Design review of the part built by this model. Coordinates are the model's own, in mm. A direction names the side the tool comes from. Round coordinates to 2 decimals unless told otherwise and drop trailing zeros.
from build123d import *

# Parameters (mm, degrees)
SKETCH_1_R      = 3.4
EXTRUDE_1_DEPTH = 1000


with BuildPart() as part:
    # Эскиз1 → Бобышка-Вытянуть1 (new body)
    with BuildSketch(Plane.XY):
        with BuildLine():
            Line((-20, 15.5), (-20, 10.25))
            Line((-20, 10.25), (-20, 5.4))
            ThreePointArc((-20, 5.4), (-19.912132034, 5.187867966), (-19.7, 5.1))
            Line((-19.7, 5.1), (-19.3, 5.1))
            ThreePointArc((-19.3, 5.1), (-19.087867966, 5.012132034), (-19, 4.8))
            Line((-19, 4.8), (-19, 4.4))
            ThreePointArc((-19, 4.4), (-18.912132034, 4.187867966), (-18.7, 4.1))
            Line((-18.7, 4.1), (-15.8, 4.1))
            ThreePointArc((-15.8, 4.1), (-15.587867966, 4.187867966), (-15.5, 4.4))
            Line((-15.5, 4.4), (-15.5, 6.3))
            ThreePointArc((-15.5, 6.3), (-15.587867966, 6.512132034), (-15.8, 6.6))
            Line((-15.8, 6.6), (-17, 6.6))
            ThreePointArc((-17, 6.6), (-17.707106781, 6.892893219), (-18, 7.6))
            Line((-18, 7.6), (-18, 9.25))
            ThreePointArc((-18, 9.25), (-17.707106781, 9.957106781), (-17, 10.25))
            Line((-17, 10.25), (-12.464213562, 10.25))
            ThreePointArc((-12.464213562, 10.25), (-12.08153013, 10.173879533), (-11.757106781, 9.957106781))
            Line((-11.757106781, 9.957106781), (-7.992893219, 6.192893219))
            ThreePointArc((-7.992893219, 6.192893219), (-7.776120467, 5.86846987), (-7.7, 5.485786438))
            Line((-7.7, 5.485786438), (-7.7, -5.485786438))
            ThreePointArc((-7.7, -5.485786438), (-7.776120467, -5.86846987), (-7.992893219, -6.192893219))
            Line((-7.992893219, -6.192893219), (-11.757106781, -9.957106781))
            ThreePointArc((-11.757106781, -9.957106781), (-12.08153013, -10.173879533), (-12.464213562, -10.25))
            Line((-12.464213562, -10.25), (-17, -10.25))
            ThreePointArc((-17, -10.25), (-17.707106781, -9.957106781), (-18, -9.25))
            Line((-18, -9.25), (-18, -7.6))
            ThreePointArc((-18, -7.6), (-17.707106781, -6.892893219), (-17, -6.6))
            Line((-17, -6.6), (-15.8, -6.6))
            ThreePointArc((-15.8, -6.6), (-15.587867966, -6.512132034), (-15.5, -6.3))
            Line((-15.5, -6.3), (-15.5, -4.4))
            ThreePointArc((-15.5, -4.4), (-15.587867966, -4.187867966), (-15.8, -4.1))
            Line((-15.8, -4.1), (-18.7, -4.1))
            ThreePointArc((-18.7, -4.1), (-18.912132034, -4.187867966), (-19, -4.4))
            Line((-19, -4.4), (-19, -4.8))
            ThreePointArc((-19, -4.8), (-19.087867966, -5.012132034), (-19.3, -5.1))
            Line((-19.3, -5.1), (-19.7, -5.1))
            ThreePointArc((-19.7, -5.1), (-19.912132034, -5.187867966), (-20, -5.4))
            Line((-20, -5.4), (-20, -10.25))
            Line((-20, -10.25), (-20, -15.5))
            ThreePointArc((-20, -15.5), (-18.681980515, -18.681980515), (-15.5, -20))
            Line((-15.5, -20), (-10.25, -20))
            Line((-10.25, -20), (0, -20))
            Line((0, -20), (10.25, -20))
            Line((10.25, -20), (15.5, -20))
            ThreePointArc((15.5, -20), (18.681980515, -18.681980515), (20, -15.5))
            Line((20, -15.5), (20, -10.25))
            Line((20, -10.25), (20, 0))
            Line((20, 0), (20, 10.25))
            Line((20, 10.25), (20, 15.5))
            ThreePointArc((20, 15.5), (18.681980515, 18.681980515), (15.5, 20))
            Line((15.5, 20), (10.25, 20))
            Line((10.25, 20), (5.4, 20))
            ThreePointArc((5.4, 20), (5.187867966, 19.912132034), (5.1, 19.7))
            Line((5.1, 19.7), (5.1, 19.3))
            ThreePointArc((5.1, 19.3), (5.012132034, 19.087867966), (4.8, 19))
            Line((4.8, 19), (4.4, 19))
            ThreePointArc((4.4, 19), (4.187867966, 18.912132034), (4.1, 18.7))
            Line((4.1, 18.7), (4.1, 15.8))
            ThreePointArc((4.1, 15.8), (4.187867966, 15.587867966), (4.4, 15.5))
            Line((4.4, 15.5), (6.3, 15.5))
            ThreePointArc((6.3, 15.5), (6.512132034, 15.587867966), (6.6, 15.8))
            Line((6.6, 15.8), (6.6, 17))
            ThreePointArc((6.6, 17), (6.892893219, 17.707106781), (7.6, 18))
            Line((7.6, 18), (9.25, 18))
            ThreePointArc((9.25, 18), (9.957106781, 17.707106781), (10.25, 17))
            Line((10.25, 17), (10.25, 12.464213562))
            ThreePointArc((10.25, 12.464213562), (10.173879533, 12.08153013), (9.957106781, 11.757106781))
            Line((9.957106781, 11.757106781), (6.192893219, 7.992893219))
            ThreePointArc((6.192893219, 7.992893219), (5.86846987, 7.776120467), (5.485786438, 7.7))
            Line((5.485786438, 7.7), (-5.485786438, 7.7))
            ThreePointArc((-5.485786438, 7.7), (-5.86846987, 7.776120467), (-6.192893219, 7.992893219))
            Line((-6.192893219, 7.992893219), (-9.957106781, 11.757106781))
            ThreePointArc((-9.957106781, 11.757106781), (-10.173879533, 12.08153013), (-10.25, 12.464213562))
            Line((-10.25, 12.464213562), (-10.25, 17))
            ThreePointArc((-10.25, 17), (-9.957106781, 17.707106781), (-9.25, 18))
            Line((-9.25, 18), (-7.6, 18))
            ThreePointArc((-7.6, 18), (-6.892893219, 17.707106781), (-6.6, 17))
            Line((-6.6, 17), (-6.6, 15.8))
            ThreePointArc((-6.6, 15.8), (-6.512132034, 15.587867966), (-6.3, 15.5))
            Line((-6.3, 15.5), (-4.4, 15.5))
            ThreePointArc((-4.4, 15.5), (-4.187867966, 15.587867966), (-4.1, 15.8))
            Line((-4.1, 15.8), (-4.1, 18.7))
            ThreePointArc((-4.1, 18.7), (-4.187867966, 18.912132034), (-4.4, 19))
            Line((-4.4, 19), (-4.8, 19))
            ThreePointArc((-4.8, 19), (-5.012132034, 19.087867966), (-5.1, 19.3))
            Line((-5.1, 19.3), (-5.1, 19.7))
            ThreePointArc((-5.1, 19.7), (-5.187867966, 19.912132034), (-5.4, 20))
            Line((-5.4, 20), (-10.25, 20))
            Line((-10.25, 20), (-15.5, 20))
            ThreePointArc((-15.5, 20), (-18.681980515, 18.681980515), (-20, 15.5))
        make_face()
        with BuildLine():
            ThreePointArc((-12.8, -11.8), (-12.092893219, -12.092893219), (-11.8, -12.8))
            Line((-11.8, -12.8), (-11.8, -17))
            ThreePointArc((-11.8, -17), (-12.092893219, -17.707106781), (-12.8, -18))
            Line((-12.8, -18), (-15.5, -18))
            ThreePointArc((-15.5, -18), (-17.267766953, -17.267766953), (-18, -15.5))
            Line((-18, -15.5), (-18, -12.8))
            ThreePointArc((-18, -12.8), (-17.707106781, -12.092893219), (-17, -11.8))
            Line((-17, -11.8), (-12.8, -11.8))
        make_face(mode=Mode.SUBTRACT)
        with BuildLine():
            Line((9.25, -18), (0, -18))
            Line((0, -18), (-9.25, -18))
            ThreePointArc((-9.25, -18), (-9.957106781, -17.707106781), (-10.25, -17))
            Line((-10.25, -17), (-10.25, -12.464213562))
            ThreePointArc((-10.25, -12.464213562), (-10.173879533, -12.08153013), (-9.957106781, -11.757106781))
            Line((-9.957106781, -11.757106781), (-6.192893219, -7.992893219))
            ThreePointArc((-6.192893219, -7.992893219), (-5.86846987, -7.776120467), (-5.485786438, -7.7))
            Line((-5.485786438, -7.7), (5.485786438, -7.7))
            ThreePointArc((5.485786438, -7.7), (5.86846987, -7.776120467), (6.192893219, -7.992893219))
            Line((6.192893219, -7.992893219), (9.957106781, -11.757106781))
            ThreePointArc((9.957106781, -11.757106781), (10.173879533, -12.08153013), (10.25, -12.464213562))
            Line((10.25, -12.464213562), (10.25, -17))
            ThreePointArc((10.25, -17), (9.957106781, -17.707106781), (9.25, -18))
        make_face(mode=Mode.SUBTRACT)
        with BuildLine():
            ThreePointArc((11.8, -12.8), (12.092893219, -12.092893219), (12.8, -11.8))
            Line((12.8, -11.8), (17, -11.8))
            ThreePointArc((17, -11.8), (17.707106781, -12.092893219), (18, -12.8))
            Line((18, -12.8), (18, -15.5))
            ThreePointArc((18, -15.5), (17.267766953, -17.267766953), (15.5, -18))
            Line((15.5, -18), (12.8, -18))
            ThreePointArc((12.8, -18), (12.092893219, -17.707106781), (11.8, -17))
            Line((11.8, -17), (11.8, -12.8))
        make_face(mode=Mode.SUBTRACT)
        Circle(SKETCH_1_R, mode=Mode.SUBTRACT)
        with BuildLine():
            ThreePointArc((-11.8, 12.8), (-12.092893219, 12.092893219), (-12.8, 11.8))
            Line((-12.8, 11.8), (-17, 11.8))
            ThreePointArc((-17, 11.8), (-17.707106781, 12.092893219), (-18, 12.8))
            Line((-18, 12.8), (-18, 15.5))
            ThreePointArc((-18, 15.5), (-17.267766953, 17.267766953), (-15.5, 18))
            Line((-15.5, 18), (-12.8, 18))
            ThreePointArc((-12.8, 18), (-12.092893219, 17.707106781), (-11.8, 17))
            Line((-11.8, 17), (-11.8, 12.8))
        make_face(mode=Mode.SUBTRACT)
        with BuildLine():
            Line((18, 9.25), (18, 0))
            Line((18, 0), (18, -9.25))
            ThreePointArc((18, -9.25), (17.707106781, -9.957106781), (17, -10.25))
            Line((17, -10.25), (12.464213562, -10.25))
            ThreePointArc((12.464213562, -10.25), (12.08153013, -10.173879533), (11.757106781, -9.957106781))
            Line((11.757106781, -9.957106781), (7.992893219, -6.192893219))
            ThreePointArc((7.992893219, -6.192893219), (7.776120467, -5.86846987), (7.7, -5.485786438))
            Line((7.7, -5.485786438), (7.7, 5.485786438))
            ThreePointArc((7.7, 5.485786438), (7.776120467, 5.86846987), (7.992893219, 6.192893219))
            Line((7.992893219, 6.192893219), (11.757106781, 9.957106781))
            ThreePointArc((11.757106781, 9.957106781), (12.08153013, 10.173879533), (12.464213562, 10.25))
            Line((12.464213562, 10.25), (17, 10.25))
            ThreePointArc((17, 10.25), (17.707106781, 9.957106781), (18, 9.25))
        make_face(mode=Mode.SUBTRACT)
        with BuildLine():
            ThreePointArc((12.8, 11.8), (12.092893219, 12.092893219), (11.8, 12.8))
            Line((11.8, 12.8), (11.8, 17))
            ThreePointArc((11.8, 17), (12.092893219, 17.707106781), (12.8, 18))
            Line((12.8, 18), (15.5, 18))
            ThreePointArc((15.5, 18), (17.267766953, 17.267766953), (18, 15.5))
            Line((18, 15.5), (18, 12.8))
            ThreePointArc((18, 12.8), (17.707106781, 12.092893219), (17, 11.8))
            Line((17, 11.8), (12.8, 11.8))
        make_face(mode=Mode.SUBTRACT)
    extrude(amount=EXTRUDE_1_DEPTH)


solid = part.part
1) Take a section at A-A on z = 939. State how many separate pieces and enclosed holes the cut face has, plus the area to 3 significant figures.
Results:
separate pieces: 1
enclosed holes: 7
area: 622 mm2
2) The part is to be moulded in two halves that separate along X. For faces 3 (the face through (0, -18, 493)), 4 (the face through (20, 0, 493)), 5 (the face through (-2, 3, 0)), say which applies: released by +X, released by -X, zero draft, split by the parting line, or undercut.
Results:
face 3: undercut
face 4: released by +X
face 5: zero draft
3) For faces 1 (the face through (-2, 3, 1000)), 2 (the face through (18, 0, 493)), list the 3-axis set-ups (+Z, -Z, +X, -X, +Y, -Y) from which the entire face can be reached by the end or side of a thin tool; tool diameter is ignored.
Results:
face 1: +Z, +X, -X, +Y, -Y
face 2: +Z, -Z
4) Clearance check with flat-ended pins moving along their axes: P1, Ø1, axis at y = 16.5, z = 622.5, coming from the +X side; P2, Ø3, axis at x = 0.5, z = 721.5, coming from the +Y side. State where each tip first meets the part, or that it passes through.
Results:
P1: stops at x = 19.97
P2: stops at y = 7.7
5) To check wall thickness, follow line 1 along Y through (x, z) = (0, 604); line 2 along X through (y, z) = (-8, 308); line 3 along Y through (x, z) = (16, 75.5). State the ranges of each line that lie inside material, in increasing order.
Results:
line 1: y = -20 to -18, -7.7 to -3.4, 3.4 to 7.7
line 2: x = -20 to -18, -9.8 to -6.2, 6.2 to 9.8, 18 to 20
line 3: y = -19.97 to -17.95, -11.8 to -10.25, 10.25 to 11.8, 17.95 to 19.97
